from build123d import *

# Parameters (mm, degrees)
INSTALLED_SPRING_STRIP_SKETCH_W = 80
INSTALLED_SPRING_STRIP_SKETCH_H = 16
INSTALLED_SPRING_STRIP_DEPTH    = 5
EYELET_CLEARANCE_1_SKETCH_R     = 2.05
EYELET_CLEARANCE_1_DEPTH        = 5.2
FLANGE_RECESS_1_1_SKETCH_R      = 3.05
FLANGE_RECESS_1_1_DEPTH         = 0.4
FLANGE_RECESS_1_2_SKETCH_R      = 3.05
FLANGE_RECESS_1_2_DEPTH         = 0.4
EYELET_CLEARANCE_2_SKETCH_R     = 2.05
EYELET_CLEARANCE_2_DEPTH        = 5.2
FLANGE_RECESS_2_1_SKETCH_R      = 3.05
FLANGE_RECESS_2_1_DEPTH         = 0.4
FLANGE_RECESS_2_2_SKETCH_R      = 3.05
FLANGE_RECESS_2_2_DEPTH         = 0.4


with BuildPart() as part:
    # Installed spring strip sketch → Installed spring strip (new body)
    with BuildSketch(Plane.XY.offset(12.5)):
        with Locations((-0.291651246, -12)):
            Rectangle(INSTALLED_SPRING_STRIP_SKETCH_W, INSTALLED_SPRING_STRIP_SKETCH_H)
    extrude(amount=INSTALLED_SPRING_STRIP_DEPTH)

    # Eyelet clearance 1 sketch → Eyelet clearance 1 (cut)
    with BuildSketch(Plane.XY.offset(12.4)):
        with Locations((-36.291651246, -12)):
            Circle(EYELET_CLEARANCE_1_SKETCH_R)
    extrude(amount=EYELET_CLEARANCE_1_DEPTH, mode=Mode.SUBTRACT)

    # Flange recess 1-1 sketch → Flange recess 1-1 (cut)
    with BuildSketch(Plane.XY.offset(12.4)):
        with Locations((-36.291651246, -12)):
            Circle(FLANGE_RECESS_1_1_SKETCH_R)
    extrude(amount=FLANGE_RECESS_1_1_DEPTH, mode=Mode.SUBTRACT)

    # Flange recess 1-2 sketch → Flange recess 1-2 (cut)
    with BuildSketch(Plane.XY.offset(17.2)):
        with Locations((-36.291651246, -12)):
            Circle(FLANGE_RECESS_1_2_SKETCH_R)
    extrude(amount=FLANGE_RECESS_1_2_DEPTH, mode=Mode.SUBTRACT)

    # Eyelet clearance 2 sketch → Eyelet clearance 2 (cut)
    with BuildSketch(Plane.XY.offset(12.4)):
        with Locations((35.708348754, -12)):
            Circle(EYELET_CLEARANCE_2_SKETCH_R)
    extrude(amount=EYELET_CLEARANCE_2_DEPTH, mode=Mode.SUBTRACT)

    # Flange recess 2-1 sketch → Flange recess 2-1 (cut)
    with BuildSketch(Plane.XY.offset(12.4)):
        with Locations((35.708348754, -12)):
            Circle(FLANGE_RECESS_2_1_SKETCH_R)
    extrude(amount=FLANGE_RECESS_2_1_DEPTH, mode=Mode.SUBTRACT)

    # Flange recess 2-2 sketch → Flange recess 2-2 (cut)
    with BuildSketch(Plane.XY.offset(17.2)):
        with Locations((35.708348754, -12)):
            Circle(FLANGE_RECESS_2_2_SKETCH_R)
    extrude(amount=FLANGE_RECESS_2_2_DEPTH, mode=Mode.SUBTRACT)


solid = part.part
Design review of the part built by this model. Coordinates are the model's own, in mm. A direction names the side the tool comes from. Give positions to 0.01 mm unless a question says otherwise; leave off trailing zeros. Loops run counter-clockwise (first coordinate to the right, second up) from the corner with the lowest first, then second, coordinate; pieces in that order, holes last. Notation, with made-up numbers: M 86.5,-25 L 92.5,-25 A15 ccw 92.5,-7 Z; hole C 21.25,9.5 d2. An arc over 180 degrees is marked long. Answer as a JSON object with one key per item and string values.
Item 1: For P1, Ø5, axis at x = 35.71, y = -12, coming from the +Z side; P2, Ø5, axis at x = 35.71, y = -12, coming from the -Z side, all flat-tipped, find the tip position at first contact; note any pin that passes through.
Output values:
{"P1": "stops at z = 17.2", "P2": "stops at z = 12.8"}
Item 2: Wall thickness on line 1 along X through (y, z) = (-12, 14.75); line 2 along X through (y, z) = (-12, 17.45); line 3 along Y through (x, z) = (35.5, 14.45): over which ranges is each line inside the solid? List them lowest first.
Output values:
{"line 1": "x = -40.29 to -38.34, -34.24 to 33.66, 37.76 to 39.71", "line 2": "x = -40.29 to -39.34, -33.24 to 32.66, 38.76 to 39.71", "line 3": "y = -20 to -14.04, -9.96 to -4"}
Item 3: We need section A-A (y = -12). State the section outline as (x, z) points, and give its area (3 significant figures).
Output values:
{"outline": "M -40.29,12.5 L -39.34,12.5 L -39.34,12.8 L -38.34,12.8 L -38.34,17.2 L -39.34,17.2 L -39.34,17.5 L -40.29,17.5 Z; M -34.24,12.8 L -33.24,12.8 L -33.24,12.5 L 32.66,12.5 L 32.66,12.8 L 33.66,12.8 L 33.66,17.2 L 32.66,17.2 L 32.66,17.5 L -33.24,17.5 L -33.24,17.2 L -34.24,17.2 Z; M 37.76,12.8 L 38.76,12.8 L 38.76,12.5 L 39.71,12.5 L 39.71,17.5 L 38.76,17.5 L 38.76,17.2 L 37.76,17.2 Z", "area": "357 mm2"}
Item 4: Machinability: for faces 1 (the face through (32.66, -11.87, 12.65)), 2 (the face through (-40.292, -12, 15)), 3 (the face through (33.46, -9.94, 17.35)), which of the approach directions +Z, -Z, +X, -X, +Y, -Y give a long, thin tool a straight path to every point of the face, cutting with its end or side? Answer none if there is none.
Output values:
{"face 1": "-Z", "face 2": "+Z, -Z, -X, +Y, -Y", "face 3": "+Z"}
Item 5: We need section B-B (z = 15.4). State the section outline as (x, y) points.
Output values:
{"outline": "M -40.29,-20 L 39.71,-20 L 39.71,-4 L -40.29,-4 Z; hole C -36.29,-12 d4.1; hole C 35.71,-12 d4.1"}
Item 6: Mouldability with a two-part tool opening along Y and no side actions: class faces 4 (the face through (-34, -13, 17.2)), 5 (the face through (-1, -12, 12.5)), 6 (the face through (-1, -20, 15)), 7 (the face through (33.66, -11.91, 14.97)) as pulls with the +Y half, pulls with the -Y half, needs draft (parallel to the pull), parting line crosses it, or undercut.
Output values:
{"face 4": "undercut", "face 5": "needs draft", "face 6": "pulls with the -Y half", "face 7": "undercut"}
